Geometry check sheet. Reference: the model listing, model coordinates, mm. A direction names the side the tool comes from. Give positions to 0.01 mm unless a question says otherwise; leave off trailing zeros. Write each loop counter-clockwise with the first axis right and the second up, starting at its lowest first coordinate (ties: lowest second). Pieces come first, ordered by that corner, then holes. Notation, with made-up numbers: M 89,-26 L 126,-26 A28 ccw 126,6 Z; hole C -39.5,65 d3. An arc over 180 degrees is marked long. One line per item, written item: value. Start each with the question number.
1. Release check for a two-part mould opening along X. For faces 1 (the face through (0, -1, 0)), 2 (the face through (0, 0.75, -0.5)), 3 (the face through (0, 1, -6)) record: pulls with the +X half, pulls with the -X half, needs draft (parallel to the pull), parting line crosses it, or undercut.
2. Cross-section at A-A on x = 0. Record the cut outline in (y, z), then the cut area to 3 significant figures.
3. Gauge pin test, flat ends, axial feed: pin 1 (1 mm diameter, centred on x = 0, y = 1.5, fed in from +Z); pin 2 (1.5 mm diameter, centred on x = -0.5, y = 1.5, fed in from -Z); pin 3 (2 mm diameter, centred on y = -1, z = -7.5, fed in from -X). Record the tip position at first contact, or that the pin passes through.
4. Cross-section at B-B on z = -4.75. Record the cut outline in (x, y).
5. Scan lines: line 1 (Z direction, x = 0.35, y = -1.05); line 2 (Z direction, x = 0.7, y = 0.2); line 3 (X direction, y = -0.05, z = -5.75). Record each from-to range of solid material in increasing order.
6. Tool access check on faces 4 (the face through (1.812, -0.571, -1.113)), 5 (the face through (1, 1, -2)), 6 (the face through (0, -0.75, -0.5)). Record the directions out of +Z, -Z, +X, -X, +Y, -Y that give a thin tool (end or side, any length) a straight path to the whole face; none if there is none.
from build123d import *

# Parameters (mm, degrees)
EXTRUDE1_DEPTH = 1
FILLET1_R      = 0.2
CHAMFER_1_SIZE = 0.2


with BuildPart() as part:
    # Sketch2 → Matrix-Rotate1 (revolve)
    with BuildSketch(Plane(origin=(0, 0, 0), x_dir=(0, 0, -1), z_dir=(1, 0, 0)), mode=Mode.PRIVATE) as matrix_rotate1_sk:
        Polygon((0, 0), (0, 1.9), (2, 1.9), (2, 1), (10, 1), (10, 0), align=None)
    revolve(matrix_rotate1_sk.sketch.rotate(Axis((0, 0, 0), (0, 0, -1)), 90), axis=Axis((0, 0, 0), (0, 0, -1)))

    # Sketch3 → Extrude1 (cut)
    with BuildSketch(Plane.XY):
        Polygon((0.866025404, 0), (0.433012702, 0.75), (-0.433012702, 0.75), (-0.866025404, 0), (-0.433012702, -0.75), (0.433012702, -0.75), align=None)
    extrude(amount=-EXTRUDE1_DEPTH, mode=Mode.SUBTRACT)

    # Fillet1
    fillet1_edges = [part.edges().sort_by_distance(p)[0] for p in [
        (-1.9, 0, 0),
    ]]
    fillet(fillet1_edges, radius=FILLET1_R)

    # 倒角1
    chamfer_1_edges = [part.edges().sort_by_distance(p)[0] for p in [
        (-1, 0, -10),
    ]]
    chamfer(chamfer_1_edges, length=CHAMFER_1_SIZE)


solid = part.part
Report:
1. face 1: needs draft
1. face 2: undercut
1. face 3: parting line crosses it
2. outline: M -1.9,-2 L -1,-2 L -1,-9.8 L -0.8,-10 L 0.8,-10 L 1,-9.8 L 1,-2 L 1.9,-2 L 1.9,-0.2 A0.2 ccw 1.7,0 L 0.75,0 L 0.75,-1 L -0.75,-1 L -0.75,0 L -1.7,0 A0.2 ccw -1.9,-0.2 Z
2. area: 22.0 mm^2
3. pin 1: stops at z = 0
3. pin 2: stops at z = -9.97
3. pin 3: stops at x = -1
4. outline: C 0,0 d2
5. line 1: z = -2 to 0
5. line 2: z = -10 to -1
5. line 3: x = -1 to 1
6. face 4: +Z, -Z
6. face 5: -Z
6. face 6: +Z
